Read the model definition and answer for the solid it produces. Units are mm, in the model's axes. Give positions to 0.01 mm unless a question says otherwise; leave off trailing zeros. Order: outer loops, then holes, each group sorted by start corner. A loop starts at its lowest first (then second) coordinate and runs counter-clockwise, first axis right, second up. Notation, with made-up numbers: (63, 47.5) - (106, 47.5) arc R18 cw to (106, 51.5) - close; hole circle Ø4 at (44.25, 69.5). An arc over 180 degrees is marked (long way). Write each question's results on one line, items separated by ' | '.
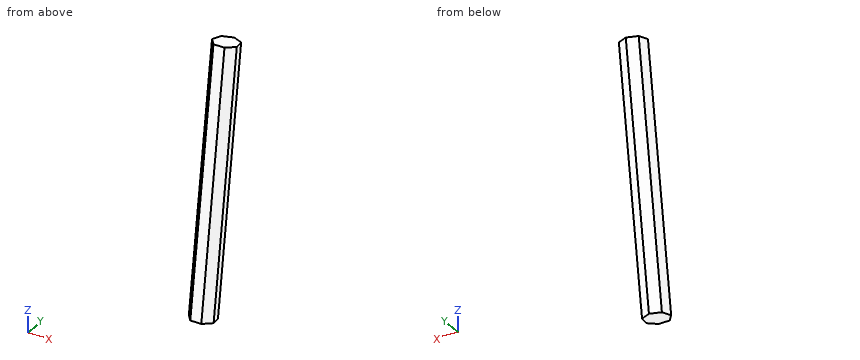
from build123d import *


with BuildPart() as part:
    # Sweep1: sweep along a path in Sketch1
    with BuildLine(Plane(origin=(0, 0, 0), x_dir=(0, 0, -1), z_dir=(1, 0, 0))) as sweep1_path:
        Line((69.282032303, 0), (0, 10))
    # Sketch2 → Sweep1 (sweep)
    with BuildSketch(Plane(origin=(0, 0, -69.282032303), x_dir=(1, 0, 0), z_dir=(0, 0.14285714285714282, 0.989743318610787))):
        Polygon((0, 3.5), (-2.736410189, 2.182214307), (-3.412247693, -0.778823269), (-1.518593087, -3.153391038), (1.518593087, -3.153391038), (3.412247693, -0.778823269), (2.736410189, 2.182214307), align=None)
    sweep(path=sweep1_path.line)


solid = part.part
(1) Each of these flat-tipped pins is pushed along its axis until it touches: pin 1 (4 mm diameter, centred on x = -1.5, z = -15, fed in from -Y); pin 2 (1.5 mm diameter, centred on x = 0.5, z = -61.5, fed in from +Y); pin 3 (2 mm diameter, centred on x = -2, y = -1.5, fed in from -Z). Where does it stop, or does it pass through?
Conclusion:
pin 1: y = 4.36 | pin 2: y = 4.74 | pin 3: z = -69.21
(2) Consider probe 1 along Y at (x, z) = (2.5, -33); probe 2 along X at (y, z) = (0, -67); probe 3 along Y at (x, z) = (-2, -28). Determine where each line is inside the solid, lowest interval first. Write a range as [from, to].
Conclusion:
probe 1: [3.29, 7.56] | probe 2: [-3.31, 3.31] | probe 3: [3.38, 8.52]
(3) Section B-B (z = -56.5) is taken. Give the vertices of the cut face in (x, y), plus the area to 3 significant figures.
Conclusion:
outline: (-3.41, 1.06) - (-1.52, -1.34) - (1.52, -1.34) - (3.41, 1.06) - (2.74, 4.05) - (0, 5.38) - (-2.74, 4.05) - close | area: 33.9 mm^2
(4) Section C-C (y = 0) is taken. Give the vertices of the cut face in (x, z).
Conclusion:
outline: (-3.41, -63.83) - (-3.23, -69.28) - (3.23, -69.28) - (3.41, -63.83) - (1.52, -47.21) - (-1.52, -47.21) - close
(5) Section A-A (y = 7.75) is taken. Give the vertices of the cut face in (x, z).
Conclusion:
outline: (-3.41, -10.14) - (-2.74, -30.86) - (0, -40.09) - (2.74, -30.86) - (3.41, -10.14) - (2.22, 0.32) - (-2.22, 0.32) - close
